Drawing for the job (mm, zero at the part's lowest x, y, z). A direction names the side the tool comes from. Round coordinates to 2 decimals unless told otherwise and drop trailing zeros. Write each loop counter-clockwise with the first axis right and the second up, starting at its lowest first coordinate (ties: lowest second). Pieces come first, ordered by that corner, then holes.
Item 1: 3-axis set-ups, long thin cutter, end or side, ignore diameter. For the marked faces 1 and 2: which of +Z, -Z, +X, -X, +Y, -Y reach the whole face in a straight line?
Item 2: Band-saw the part on A-A, the plane z = 1. Write the cut outline in (x, y).
Item 3: Band-saw the part on C-C, the plane x = 20.5. Write the cut outline in (y, z), then the cut area to 3 significant figures.
Item 4: Wall check: probe 1 along X at (y, z) = (5, 1); probe 2 along Z at (x, y) = (21, 2.5); probe 3 along X at (y, z) = (2.75, 1.75). Give the ranges that are in metal, low to high.
Item 5: Band-saw the part on B-B, the plane y = 6. Write the cut outline in (x, z).
Item 6: Drop flat-ended pins along their axis: pin 1 Ø1.5 at (x, y) = (62, 5.5) entering from -Z; pin 2 Ø4 at (x, y) = (31, 5) entering from +Z; pin 3 Ø5 at (x, z) = (36, 10.5) entering from +Y. Give the stop position or say it passes through.
Item 7: Band-saw the part on D-D, the plane z = 11. Write the cut outline in (x, y), then the cut area to 3 significant figures.
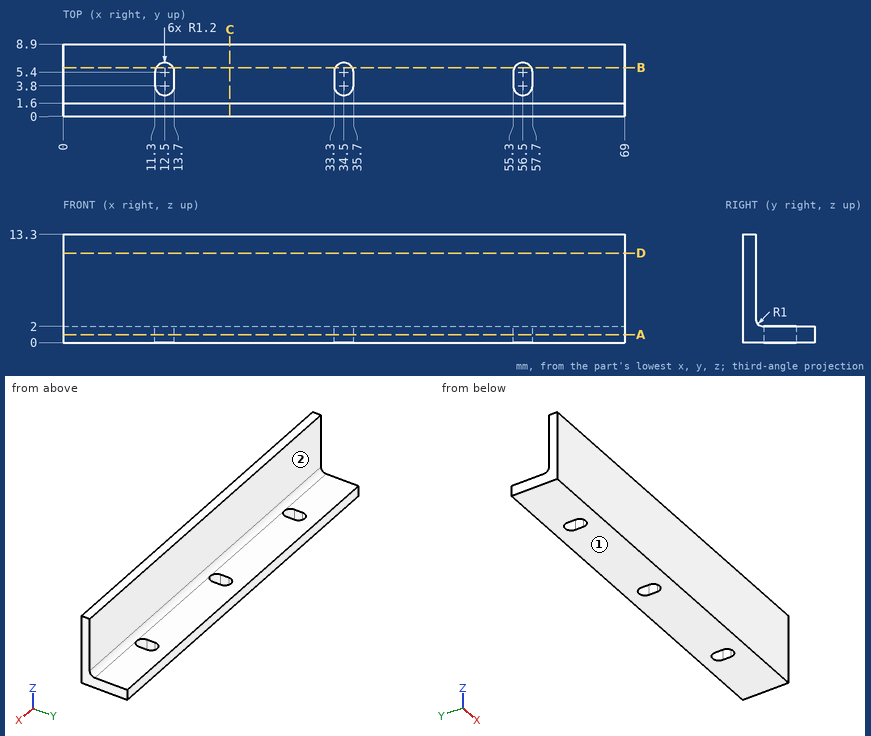
Results:
1. face 1: -Z, +X, -X, +Y, -Y
1. face 2: +Z, +X, -X, +Y
2. outline: (0, 0) - (69, 0) - (69, 8.9) - (0, 8.9) - close; hole (11.3, 3.8) arc R1.2 ccw to (13.7, 3.8) - (13.7, 5.4) arc R1.2 ccw to (11.3, 5.4) - close; hole (33.3, 3.8) arc R1.2 ccw to (35.7, 3.8) - (35.7, 5.4) arc R1.2 ccw to (33.3, 5.4) - close; hole (55.3, 3.8) arc R1.2 ccw to (57.7, 3.8) - (57.7, 5.4) arc R1.2 ccw to (55.3, 5.4) - close
3. outline: (0, 0) - (8.9, 0) - (8.9, 2) - (2.6, 2) arc R1 cw to (1.6, 3) - (1.6, 13.3) - (0, 13.3) - close
3. area: 36.1 mm2
4. probe 1: x = 0 to 11.3, 13.7 to 33.3, 35.7 to 55.3, 57.7 to 69
4. probe 2: z = 0 to 2.01
4. probe 3: x = 0 to 11.92, 13.08 to 33.92, 35.08 to 55.92, 57.08 to 69
5. outline: (0, 0) - (11.46, 0) - (11.46, 2) - (0, 2) - close; (13.54, 0) - (33.46, 0) - (33.46, 2) - (13.54, 2) - close; (35.54, 0) - (55.46, 0) - (55.46, 2) - (35.54, 2) - close; (57.54, 0) - (69, 0) - (69, 2) - (57.54, 2) - close
6. pin 1: stops at z = 0
6. pin 2: stops at z = 2
6. pin 3: stops at y = 1.6
7. outline: (0, 0) - (69, 0) - (69, 1.6) - (0, 1.6) - close
7. area: 110 mm2
